The model under review builds one solid part; all positions refer to its coordinate system, in mm. Coordinates: 2 decimals unless noted, no trailing zeros. Loops run counter-clockwise (first coordinate to the right, second up) from the corner with the lowest first, then second, coordinate; pieces in that order, holes last. Notation, with made-up numbers: M -24.75,34 L 1.25,34 A34 ccw 1.25,66 Z; hole C 1.5,-31 d10. An arc over 180 degrees is marked long. Use CSV: the item, a comma, the result in double quotes. Start each with the question number.
1. For L1, parallel to X at y = -5335.5, z = -1; L2, parallel to Y at x = -268.5, z = -6.5 (3 decimals); L3, parallel to X at y = -5409, z = -3, list the stretches that pass through material, from the lowest coordinate up.
2. Add section B-B, the plane y = -5403.5. Write out the cut boundary in (x, z), then the cut area to 3 significant figures.
3. Add section A-A, the plane x = -270.5. Write out the cut boundary in (y, z) (3 decimals), then the cut area to 3 significant figures.
4. Add section C-C, the plane z = -4.75. State how many separate pieces and enclosed holes the cut face has, then the cut area to 3 significant figures.
from build123d import *

# Parameters (mm, degrees)
SKETCH2_W          = 740.41
SKETCH2_H          = 187.325
EXTRUDE1_DEPTH     = 21.59
SKETCH3_R          = 1.5875
CUT_EXTRUDE1_DEPTH = 21.59


with BuildPart() as part:
    # Sketch2 → Extrude1 (new body)
    with BuildSketch(Plane.XY):
        with Locations((-233.045, -5408.6125)):
            Rectangle(SKETCH2_W, SKETCH2_H)
    extrude(amount=-EXTRUDE1_DEPTH)

    # Sketch3 → Cut-Extrude1 (cut)
    with BuildSketch(Plane.XY):
        with Locations((-429.895, -5484.0124)):
            Circle(SKETCH3_R)
        with Locations((-379.095, -5484.0124)):
            Circle(SKETCH3_R)
        with Locations((-86.995, -5484.0124)):
            Circle(SKETCH3_R)
        with Locations((-36.195, -5484.0124)):
            Circle(SKETCH3_R)
        with BuildLine():
            Line((-302.10125, -5335.905), (-302.10125, -5432.425))
            ThreePointArc((-302.10125, -5432.425), (-301.17131403, -5434.67006403), (-298.92625, -5435.6))
            Line((-298.92625, -5435.6), (-167.16375, -5435.6))
            ThreePointArc((-167.16375, -5435.6), (-164.91868597, -5434.67006403), (-163.98875, -5432.425))
            Line((-163.98875, -5432.425), (-163.98875, -5335.905))
            ThreePointArc((-163.98875, -5335.905), (-164.91868597, -5333.65993597), (-167.16375, -5332.73))
            Line((-167.16375, -5332.73), (-298.92625, -5332.73))
            ThreePointArc((-298.92625, -5332.73), (-301.17131403, -5333.65993597), (-302.10125, -5335.905))
        make_face()
        with BuildLine():
            Line((-354.2665, -5334), (-354.2665, -5341.9375))
            ThreePointArc((-354.2665, -5341.9375), (-356.888919435, -5348.268580565), (-363.22, -5350.891))
            Line((-363.22, -5350.891), (-433.07, -5350.891))
            ThreePointArc((-433.07, -5350.891), (-439.401080565, -5348.268580565), (-442.0235, -5341.9375))
            Line((-442.0235, -5341.9375), (-442.0235, -5334))
            ThreePointArc((-442.0235, -5334), (-440.79598452, -5331.03651548), (-437.8325, -5329.809))
            Line((-437.8325, -5329.809), (-358.4575, -5329.809))
            ThreePointArc((-358.4575, -5329.809), (-355.49401548, -5331.03651548), (-354.2665, -5334))
        make_face()
        with BuildLine():
            Line((-102.87, -5350.891), (-33.02, -5350.891))
            ThreePointArc((-33.02, -5350.891), (-26.688919435, -5348.268580565), (-24.0665, -5341.9375))
            Line((-24.0665, -5341.9375), (-24.0665, -5334))
            ThreePointArc((-24.0665, -5334), (-25.29401548, -5331.03651548), (-28.2575, -5329.809))
            Line((-28.2575, -5329.809), (-107.6325, -5329.809))
            ThreePointArc((-107.6325, -5329.809), (-110.59598452, -5331.03651548), (-111.8235, -5334))
            Line((-111.8235, -5334), (-111.8235, -5341.9375))
            ThreePointArc((-111.8235, -5341.9375), (-109.201080565, -5348.268580565), (-102.87, -5350.891))
        make_face()
    extrude(amount=-CUT_EXTRUDE1_DEPTH, mode=Mode.SUBTRACT)


solid = part.part
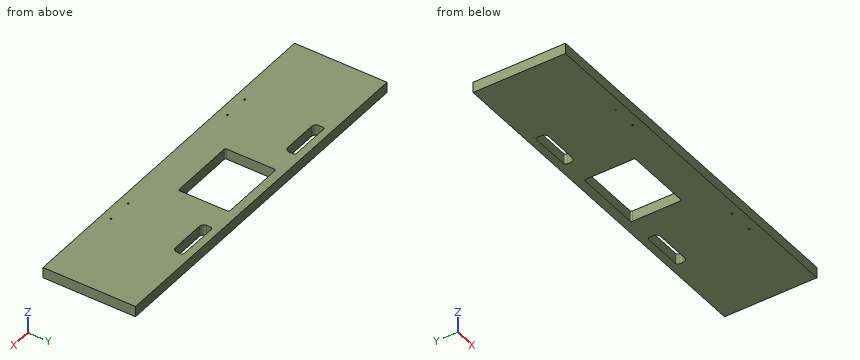
Computed:
1,L1,"x = -603.25 to -442.02, -354.27 to -302.08, -164.01 to -111.82, -24.07 to 137.16"
1,L2,"y = -5502.275 to -5435.6, -5332.73 to -5314.95"
1,L3,"x = -603.25 to -302.1, -163.99 to 137.16"
2,outline,"M -603.25,-21.59 L -302.1,-21.59 L -302.1,0 L -603.25,0 Z; M -163.99,-21.59 L 137.16,-21.59 L 137.16,0 L -163.99,0 Z"
2,area,"13,000 mm^2"
3,outline,"M -5502.275,-21.59 L -5435.6,-21.59 L -5435.6,0 L -5502.275,0 Z; M -5332.73,-21.59 L -5314.95,-21.59 L -5314.95,0 L -5332.73,0 Z"
3,area,"1,820 mm^2"
4,separate pieces,"1"
4,enclosed holes,"7"
4,area,"121,000 mm^2"
